```python
from build123d import *

# Parameters (mm, degrees)
SKETCH_1_R          = 6.75
EXTRUDE_1_DEPTH     = 21
SKETCH_2_R          = 5.5
CUT_EXTRUDE_1_DEPTH = 0.2
CUT_EXTRUDE_2_DEPTH = 0.2
FILLET_1_R          = 0.25
SKETCH_5_R          = 0.6
EXTRUDE_2_DEPTH     = 2
WRAP_START          = 10.027777778
WRAP_2_DEPTH        = 3.263888889
WRAP_START_2        = 17.527777778
WRAP_2_2_DEPTH      = 3.263888889


# Read off the part's stored shape, not the designer's step: 包覆2
with BuildPart() as part:
    # 草图1 → 凸台-拉伸1 (new body)
    with BuildSketch(Plane.XY):
        with Locations(Location((0, 0, 0), (0, 0, 180))):
            Circle(SKETCH_1_R)
    extrude(amount=EXTRUDE_1_DEPTH)

    # 草图2 → 切除-拉伸1 (cut)
    with BuildSketch(Plane.XY.offset(21)):
        Circle(SKETCH_2_R)
    extrude(amount=-CUT_EXTRUDE_1_DEPTH, mode=Mode.SUBTRACT)

    # 草图3 → 切除-拉伸2 (cut)
    with BuildSketch(Plane.XY.offset(20.8)):
        with BuildLine():
            Line((-0.04330127, 0.025), (-0.028867513, 0.05))
            Line((-0.028867513, 0.05), (-5.499772723, 0.05))
            ThreePointArc((-5.499772723, 0.05), (-5.5, 0), (-5.499772723, -0.05))
            Line((-5.499772723, -0.05), (-0.028867513, -0.05))
            Line((-0.028867513, -0.05), (-0.04330127, -0.025))
            Line((-0.04330127, -0.025), (0, 0))
            Line((0, 0), (-0.04330127, 0.025))
        make_face()
        with BuildLine():
            Line((0.04330127, -0.025), (0, 0))
            Line((0, 0), (0, -0.05))
            Line((0, -0.05), (-0.028867513, -0.05))
            Line((-0.028867513, -0.05), (2.706585091, -4.787942893))
            ThreePointArc((2.706585091, -4.787942893), (2.75, -4.763139721), (2.793187631, -4.737942893))
            Line((2.793187631, -4.737942893), (0.057735027, 0))
            Line((0.057735027, 0), (0.04330127, -0.025))
        make_face()
        with BuildLine():
            Line((-0.028867513, 0.05), (0, 0.05))
            Line((0, 0.05), (0, 0))
            Line((0, 0), (0.04330127, 0.025))
            Line((0.04330127, 0.025), (0.057735027, 0))
            Line((0.057735027, 0), (2.793187631, 4.737942893))
            ThreePointArc((2.793187631, 4.737942893), (2.75, 4.763139721), (2.706585091, 4.787942893))
            Line((2.706585091, 4.787942893), (-0.028867513, 0.05))
        make_face()
        Polygon((0, 0), (0, 0.05), (-0.028867513, 0.05), (-0.04330127, 0.025), align=None)
        Polygon((0, -0.05), (0, 0), (-0.04330127, -0.025), (-0.028867513, -0.05), align=None)
        Polygon((0.04330127, 0.025), (0, 0), (0.04330127, -0.025), (0.057735027, 0), align=None)
    extrude(amount=-CUT_EXTRUDE_2_DEPTH, mode=Mode.SUBTRACT)

    # 草图4 → 切除-旋转1 (revolve, cut)
    with BuildSketch(Plane(origin=(0, 0, 0), x_dir=(1, 0, 0), z_dir=(0, 1, 0))):
        with BuildLine():
            Line((-6.818421305, -2.223982894), (-6.818421305, -6.342581877))
            ThreePointArc((-6.818421305, -6.342581877), (-6, -4.283282386), (-6.818421305, -2.223982894))
        make_face()
    revolve(axis=Axis((0, 0, 0), (0, 0, 1)), mode=Mode.SUBTRACT)

    # 圆角1
    fillet_1_edges = [part.edges().sort_by_distance(p)[0] for p in [
        (6.75, 0, 6.267595869),
        (6.75, 0, 2.298968902),
    ]]
    fillet(fillet_1_edges, radius=FILLET_1_R)

    # 草图5 → 凸台-拉伸2 (add)
    with BuildSketch(Plane(origin=(0, 0, 0), x_dir=(-1, 0, 0), z_dir=(0, 0, -1))):
        with Locations(Location((2.54, 0, 0), (0, 0, 180))):
            Circle(SKETCH_5_R)
        with Locations(Location((-2.54, 0, 0), (0, 0, 180))):
            Circle(SKETCH_5_R)
    extrude(amount=EXTRUDE_2_DEPTH)

    # 包覆2 outline → 包覆2 (cut)
    with BuildSketch(Plane.XY.offset(WRAP_START)):
        with BuildLine():
            Line((6.661018662, 1.092396624), (5.674201083, 0.930560087))
            ThreePointArc((5.674201083, 0.930560087), (5.687885367, 0.842887927), (5.700215109, 0.755015037))
            Line((5.700215109, 0.755015037), (6.691556868, 0.886322))
            ThreePointArc((6.691556868, 0.886322), (6.677082822, 0.989477131), (6.661018662, 1.092396624))
        make_face()
    extrude(amount=WRAP_2_DEPTH, mode=Mode.SUBTRACT)

    # Wrap 2 2 outline → Wrap 2 2 (cut)
    with BuildSketch(Plane.XY.offset(WRAP_START_2)):
        with BuildLine():
            Line((6.661018662, 1.092396624), (5.674201083, 0.930560087))
            ThreePointArc((5.674201083, 0.930560087), (5.687885367, 0.842887927), (5.700215109, 0.755015037))
            Line((5.700215109, 0.755015037), (6.691556868, 0.886322))
            ThreePointArc((6.691556868, 0.886322), (6.677082822, 0.989477131), (6.661018662, 1.092396624))
        make_face()
    extrude(amount=WRAP_2_2_DEPTH, mode=Mode.SUBTRACT)


solid = part.part
```
Part model, mm, in its own coordinate system. A direction names the side the tool comes from. Round coordinates to 2 decimals unless told otherwise and drop trailing zeros. Loops run counter-clockwise (first coordinate to the right, second up) from the corner with the lowest first, then second, coordinate; pieces in that order, holes last.
1. Flat gauge pins, fed straight in: pin 1 (3 mm diameter, centred on x = 2.5, y = 3, fed in from -Z); pin 2 (1.5 mm diameter, centred on x = 3.5, z = 9.5, fed in from +Y); pin 3 (2 mm diameter, centred on y = 4.5, z = 3.5, fed in from +X). Where does each tip first touch, or does it go through?
Solutions:
pin 1: stops at z = 0
pin 2: stops at y = 6.16
pin 3: stops at x = 5.15
2. Two-plate mould, pull along X, no slides. Class faces 1 (the face through (6.19, 0.82, 19.14)), 2 (the face through (-2.5, 0, -2)), 3 (the face through (6.17, 1.01, 19.14)): pulls with the +X half, pulls with the -X half, needs draft (parallel to the pull), parting line crosses it, or undercut.
Solutions:
face 1: undercut
face 2: needs draft
face 3: pulls with the +X half
3. Slice it at A-A (z = 11). Give the cut face in (x, y), and give its area (3 significant figures).
Solutions:
outline: (5.67, 0.93) - (6.66, 1.09) arc R6.75 ccw (long way) to (6.69, 0.89) - (5.7, 0.76) arc R5.75 ccw to start
area: 143 mm2
4. 3-axis set-ups, long thin cutter, end or side, ignore diameter. For faces 4 (the face through (3, 0, 20.8)), 5 (the face through (-3.14, -0.03, -0.99)), 6 (the face through (6.17, 1.01, 11.64)), 7 (the face through (6.19, 0.82, 11.64)), 8 (the face through (6, 0, 21)): which of +Z, -Z, +X, -X, +Y, -Y reach the whole face in a straight line?
Solutions:
face 4: +Z
face 5: -Z
face 6: +X
face 7: none
face 8: +Z, +X, -X, +Y, -Y
5. Drill centre lines: line 1 along Y through (x, z) = (0, 20.95); line 2 along Z through (x, y) = (-3.25, -3.75); line 3 along Z through (x, y) = (-2.5, -0.25). Where is each one in solid material? Low to high.
Solutions:
line 1: y = -6.75 to -5.5, 5.5 to 6.75
line 2: z = 0 to 20.8
line 3: z = -2 to 20.8
6. Slice it at B-B (z = 17.25). Give the cut face in (x, y), and give its area (3 significant figures).
Solutions:
outline: circle Ø13.5 at (0, 0)
area: 143 mm2
